```python
from build123d import *

# Parameters (mm, degrees)
F0_R     = 28.067
F0_R_2   = 40.894
F1_DEPTH = 11.43


with BuildPart() as f1:
    # F0 (on Top) → F1 (new body, symmetric)
    with BuildSketch(Plane.XY):
        with BuildLine():
            ThreePointArc((-39.96043, -56.685273), (-35.633978, -47.925871), (-34.145784, -38.270273))
            ThreePointArc((-34.145784, -38.270273), (-55.239867, -8.13875), (-90.770633, -17.648411))
            ThreePointArc((-90.770633, -17.648411), (-85.750117, -63.699325), (-39.96043, -56.685273))
        make_face()
        with Locations((-66.213284, -38.270273)):
            Circle(F0_R, mode=Mode.SUBTRACT)
        with BuildLine():
            ThreePointArc((-90.770633, -17.648411), (-55.239867, -8.13875), (-34.145784, -38.270273))
            ThreePointArc((-34.145784, -38.270273), (-35.633978, -47.925871), (-39.96043, -56.685273))
            add(Edge.make_bspline(
                [(-39.96043, -56.685273), (-15.055393, -29.895963), (28.272031, -65.460931), (62.38831, -69.848491)],
                knots=[0, 0, 0, 0, 103.191739, 103.191739, 103.191739, 103.191739], degree=3))
            ThreePointArc((62.38831, -69.848491), (36.17807, -34.065405), (70.790123, -6.327134))
            add(Edge.make_bspline(
                [(70.790123, -6.327134), (35.137381, 1.846606), (44.273835, 57.15174), (31.015434, 88.891084)],
                knots=[0, 0, 0, 0, 103.191739, 103.191739, 103.191739, 103.191739], degree=3))
            ThreePointArc((31.015434, 88.891084), (32.459077, 83.49723), (32.945204, 77.934727))
            ThreePointArc((32.945204, 77.934727), (7.805363, 46.624472), (-28.196581, 64.406589))
            add(Edge.make_bspline(
                [(-28.196581, 64.406589), (-17.448877, 29.443539), (-69.912755, 9.703373), (-90.770633, -17.648411)],
                knots=[0, 0, 0, 0, 103.191739, 103.191739, 103.191739, 103.191739], degree=3))
        make_face()
        with Locations((0.877704, 0.464727)):
            Circle(F0_R_2, mode=Mode.SUBTRACT)
        with BuildLine():
            ThreePointArc((31.015434, 88.891084), (-11.376085, 107.568647), (-28.196581, 64.406589))
            ThreePointArc((-28.196581, 64.406589), (7.805363, 46.624472), (32.945204, 77.934727))
            ThreePointArc((32.945204, 77.934727), (32.459077, 83.49723), (31.015434, 88.891084))
        make_face()
        with Locations((0.877704, 77.934727)):
            Circle(F0_R, mode=Mode.SUBTRACT)
        with BuildLine():
            ThreePointArc((70.790123, -6.327134), (36.17807, -34.065405), (62.38831, -69.848491))
            ThreePointArc((62.38831, -69.848491), (88.576647, -62.839292), (100.036192, -38.270273))
            ThreePointArc((100.036192, -38.270273), (91.620339, -16.615616), (70.790123, -6.327134))
        make_face()
        with Locations((67.968692, -38.270273)):
            Circle(F0_R, mode=Mode.SUBTRACT)
    extrude(amount=F1_DEPTH, both=True)


solid = f1.part
```
CAD build for the part. Positions are in the model's coordinates, mm. Give positions to 0.01 mm unless a question says otherwise; leave off trailing zeros. Write each loop counter-clockwise with the first axis right and the second up, starting at its lowest first coordinate (ties: lowest second). Pieces come first, ordered by that corner, then holes. Notation, with made-up numbers: (8.5, -12.75) -> (36.5, -12.75) arc R22 cw to (36.5, 14.25) -> close; hole circle Ø3 at (4.25, 50.5). An arc over 180 degrees is marked (long way). Write each question's results on one line, items separated by ' | '.
1. Cut at C-C, the plane y = -43.5. Write the cut outline in (x, z).
Geometry check:
outline: (-97.85, -11.43) -> (-93.79, -11.43) -> (-93.79, 11.43) -> (-97.85, 11.43) -> close; (-38.64, -11.43) -> (40.39, -11.43) -> (40.39, 11.43) -> (-38.64, 11.43) -> close; (95.54, -11.43) -> (99.61, -11.43) -> (99.61, 11.43) -> (95.54, 11.43) -> close
2. Cut at D-D, the plane z = -5.5. Give the number of separate pieces and of enclosed holes in the cut face, then the cut area to 3 significant figures.
Geometry check:
separate pieces: 1 | enclosed holes: 4 | area: 6,460 mm²
3. Drop flat-ended pins along their axis: P1, Ø12, axis at y = 69.5, z = -7.5, coming from the -X side; P2, Ø1, axis at x = 62, z = -1, coming from the -Y side; P3, Ø2, axis at y = 41, z = 3, coming from the +X side; P4, Ø2, axis at x = 23, y = 34.5, coming from the -Z side. Give the stop position or say it passes through.
Geometry check:
P1: x = -31.1 | P2: y = -69.87 | P3: x = 41.12 | P4: z = -11.43
4. Cut at B-B, the plane y = -22. Write the cut outline in (x, z).
Geometry check:
outline: (-93.85, -11.43) -> (-89.08, -11.43) -> (-89.08, 11.43) -> (-93.85, 11.43) -> close; (-43.34, -11.43) -> (-33.29, -11.43) -> (-33.29, 11.43) -> (-43.34, 11.43) -> close; (35.05, -11.43) -> (45.1, -11.43) -> (45.1, 11.43) -> (35.05, 11.43) -> close; (90.84, -11.43) -> (95.6, -11.43) -> (95.6, 11.43) -> (90.84, 11.43) -> close
5. Cut at A-A, the plane x = 75.5. Write the cut outline in (y, z), then the cut area to 3 significant figures.
Geometry check:
outline: (-69.44, -11.43) -> (-65.31, -11.43) -> (-65.31, 11.43) -> (-69.44, 11.43) -> close; (-11.23, -11.43) -> (-7.1, -11.43) -> (-7.1, 11.43) -> (-11.23, 11.43) -> close | area: 189 mm²
6. Wall check: probe 1 along Y at (x, z) = (-2, -2.75); probe 2 along Y at (x, z) = (0, -4.25); probe 3 along Y at (x, z) = (-76, 5.25). Give the ranges that are in metal, low to high. Write a range as [from, to].
Geometry check:
probe 1: [-48.72, -40.33], [41.26, 50.02], [105.85, 109.87] | probe 2: [-49.23, -40.42], [41.35, 49.88], [105.99, 109.99] | probe 3: [-68.81, -64.58], [-11.96, -2.63]
